```python
from build123d import *

# Parameters (mm, degrees)
SKETCH1_W                       = 344.6280001
SKETCH1_H                       = 182.714000078
BASE_FLANGE1_DEPTH              = 2.286
EDGE_FLANGE1_STRIP_W            = 13.9065
EDGE_FLANGE1_STRIP_H            = 2.286
EDGE_FLANGE1_STRIP_CUT_DEPTH    = 182.714000078
EDGE_FLANGE1_STRIP_2_W          = 13.9065
EDGE_FLANGE1_STRIP_2_H          = 2.286
EDGE_FLANGE1_STRIP_CUT_2_DEPTH  = 182.714000078
EDGE_FLANGE1_DEPTH              = 182.714000078
EDGE_FLANGE1_BEND_DEPTH         = 182.714000078
EDGE_FLANGE2_STRIP_W            = 13.9065
EDGE_FLANGE2_STRIP_H            = 2.286
EDGE_FLANGE2_STRIP_CUT_DEPTH    = 339.8655001
EDGE_FLANGE2_DEPTH              = 339.8655001
SKETCH17_W                      = 38.1
SKETCH17_H                      = 31.75
CUT_EXTRUDE1_DEPTH              = 200.412142834
FILLET1_R                       = 2.54
F_11_0_191_DIAMETER_HOLE1_D     = 4.8514
F_11_0_191_DIAMETER_HOLE1_DEPTH = 349.2000001
F_11_0_191_DIAMETER_HOLE1_TIP   = 1.457507604


# Sheet-metal steps are written as plain solids
with BuildPart() as part:
    # Sketch1 → Base-Flange1 (new body)
    with BuildSketch(Plane.XY):
        Rectangle(SKETCH1_W, SKETCH1_H)
    extrude(amount=-BASE_FLANGE1_DEPTH)

    # Edge-Flange1 strip (across the edge) → Edge-Flange1 strip cut (cut)
    with BuildSketch(Plane(origin=(172.31400005, -91.357000039, 0), x_dir=(-1, 0, 0), z_dir=(0, 1, 0))):
        with Locations((-4.572, -1.143)):
            Rectangle(EDGE_FLANGE1_STRIP_W, EDGE_FLANGE1_STRIP_H)
    extrude(amount=EDGE_FLANGE1_STRIP_CUT_DEPTH, mode=Mode.SUBTRACT)

    # Edge-Flange1 strip 2 (across the edge) → Edge-Flange1 strip cut 2 (cut)
    with BuildSketch(Plane(origin=(-172.31400005, 91.357000039, 0), x_dir=(1, 0, 0), z_dir=(0, -1, 0))):
        with Locations((-4.572, -1.143)):
            Rectangle(EDGE_FLANGE1_STRIP_2_W, EDGE_FLANGE1_STRIP_2_H)
    extrude(amount=EDGE_FLANGE1_STRIP_CUT_2_DEPTH, mode=Mode.SUBTRACT)

    # Edge-Flange1 section (across the edge) → Edge-Flange1 (add)
    with BuildSketch(Plane(origin=(172.31400005, -91.357000039, 0), x_dir=(-1, 0, 0), z_dir=(0, 1, 0))):
        with BuildLine():
            Line((-2.286, 2.38125), (-2.286, 20.32))
            Line((-2.286, 20.32), (0, 20.32))
            Line((0, 20.32), (0, 2.38125))
            ThreePointArc((0, 2.38125), (0.697451977, 0.697451977), (2.38125, 0))
            Line((2.38125, 0), (2.38125, -2.286))
            ThreePointArc((2.38125, -2.286), (-0.918994124, -0.918994124), (-2.286, 2.38125))
        make_face()
    extrude(amount=EDGE_FLANGE1_DEPTH)

    # Edge-Flange1 section 2 (across the edge) → Edge-Flange1 bend (add)
    with BuildSketch(Plane(origin=(-172.31400005, 91.357000039, 0), x_dir=(1, 0, 0), z_dir=(0, -1, 0))):
        with BuildLine():
            Line((-2.286, 2.38125), (-2.286, 20.32))
            Line((-2.286, 20.32), (0, 20.32))
            Line((0, 20.32), (0, 2.38125))
            ThreePointArc((0, 2.38125), (0.697451977, 0.697451977), (2.38125, 0))
            Line((2.38125, 0), (2.38125, -2.286))
            ThreePointArc((2.38125, -2.286), (-0.918994124, -0.918994124), (-2.286, 2.38125))
        make_face()
    extrude(amount=EDGE_FLANGE1_BEND_DEPTH)

    # Edge-Flange2 strip (across the edge) → Edge-Flange2 strip cut (cut)
    with BuildSketch(Plane(origin=(169.93275005, -91.357000039, -2.286), x_dir=(0, 1, 0), z_dir=(-1, 0, 0))):
        with Locations((-4.572, -1.143)):
            Rectangle(EDGE_FLANGE2_STRIP_W, EDGE_FLANGE2_STRIP_H)
    extrude(amount=EDGE_FLANGE2_STRIP_CUT_DEPTH, mode=Mode.SUBTRACT)

    # Edge-Flange2 section (across the edge) → Edge-Flange2 (add)
    with BuildSketch(Plane(origin=(169.93275005, -91.357000039, -2.286), x_dir=(0, 1, 0), z_dir=(-1, 0, 0))):
        with BuildLine():
            Line((-2.286, 2.38125), (-2.286, 19.05))
            Line((-2.286, 19.05), (0, 19.05))
            Line((0, 19.05), (0, 2.38125))
            ThreePointArc((0, 2.38125), (0.697451977, 0.697451977), (2.38125, 0))
            Line((2.38125, 0), (2.38125, -2.286))
            ThreePointArc((2.38125, -2.286), (-0.918994124, -0.918994124), (-2.286, 2.38125))
        make_face()
    extrude(amount=EDGE_FLANGE2_DEPTH)

    # Sketch17 → Cut-Extrude1 (cut, through all)
    with BuildSketch(Plane(origin=(0, 0, -2.286), x_dir=(-1, 0, 0), z_dir=(0, 0, -1))):
        with Locations((145.80275005, 75.482000039)):
            Rectangle(SKETCH17_W, SKETCH17_H)
    extrude(amount=-CUT_EXTRUDE1_DEPTH, mode=Mode.SUBTRACT)

    # Fillet1
    fillet1_edges = [part.edges().sort_by_distance(p)[0] for p in [
        (169.93275005, -92.500000039, -21.336),
        (-169.93275005, -92.500000039, -21.336),
        (-126.75275005, 91.357000039, -1.143),
        (-164.85275005, 91.357000039, -1.143),
        (-164.85275005, 59.607000039, -1.143),
        (-126.75275005, 59.607000039, -1.143),
        (173.45700005, -91.357000039, 20.32),
        (173.45700005, 91.357000039, 20.32),
        (-173.45700005, 91.357000039, 20.32),
        (-173.45700005, -91.357000039, 20.32),
    ]]
    fillet(fillet1_edges, radius=FILLET1_R)

    # #11 (0.191) Diameter Hole1
    with Locations(Plane.ZY.offset(174.60000005)):
        with Locations((10.080625, -73.742999961), (10.080625, 78.657000039), (10.080625, 53.257000039), (10.080625, 27.857000039), (10.080625, 2.457000039), (10.080625, -22.942999961), (10.080625, -48.342999961)):
            Hole(F_11_0_191_DIAMETER_HOLE1_D / 2, depth=F_11_0_191_DIAMETER_HOLE1_DEPTH)
            with Locations((0, 0, -(F_11_0_191_DIAMETER_HOLE1_DEPTH + F_11_0_191_DIAMETER_HOLE1_TIP / 2))):  # 118° drill point
                Cone(0, F_11_0_191_DIAMETER_HOLE1_D / 2, F_11_0_191_DIAMETER_HOLE1_TIP, mode=Mode.SUBTRACT)


solid = part.part
```
Can you work these out from the model? Positions are in its coordinate system, mm. A direction names the side the tool comes from. Round coordinates to 2 decimals unless told otherwise and drop trailing zeros. Loops run counter-clockwise (first coordinate to the right, second up) from the corner with the lowest first, then second, coordinate; pieces in that order, holes last. Notation, with made-up numbers: M -39,49 L 13,49 A34 cw 13,80 Z; hole C -29.75,85.5 d2. An arc over 180 degrees is marked long. Write item = value, one per line. Start each with the question number.
(1) Suppose I cut it at B-B on x = 34. Write out the boundary of the cut face in (y, z), plus the area to 3 significant figures.
(2) If we mould it in two halves opening along X, with no side actions, what happens to faces 4 (the face through (-172.314, 1, 13)), 5 (the face through (-174.6, 1, 13)), 6 (the face through (174.6, -1, 11))? For each: released by +X, released by -X, zero draft, split by the parting line, or undercut.
(3) I need wall thicknesses on line 1 along X through (y, z) = (71, 7.5); line 2 along Z through (x, y) = (-147, 5); line 3 along X through (y, z) = (-10, 0.5). Which ranges of each line are inside material? Lowest first, please.
(4) Suppose I cut it at C-C on y = -12. Write out the boundary of the cut face in (x, z), plus the area to 3 significant figures.
(5) I'm going to push flat-ended pins straight in: P1, Ø8, axis at y = -22.94, z = 10.08, coming from the -X side; P2, Ø0.5, axis at y = -90.5, z = -0.5, coming from the +X side; P3, Ø4, axis at x = 105, y = 10.5, coming from the +Z side; P4, Ø12, axis at x = -118.5, y = 32, coming from the -Z side. Where does each tip first touch, or does it pass through?
(6) Suppose I cut it at D-D on z = -15.5. Write out the boundary of the cut face in (x, y).
(7) Suppose I cut it at A-A on y = 69. Write out the boundary of the cut face in (x, z), plus the area to 3 significant figures.
(8) Which directions (+Z, -Z, +X, -X, +Y, -Y) give clear straight access to the entire face, cutting with the end or side of a thin tool? Please do faces 1 (the face through (172.314, -1, 11)), 2 (the face through (26, 91.357, -1)), 3 (the face through (2, -91.357, -13)).
Answer block:
q1.outline = M -93.64,-21.34 L -91.36,-21.34 L -91.36,-4.67 A2.38 cw -88.98,-2.29 L 91.36,-2.29 L 91.36,0 L -88.98,0 A4.67 ccw -93.64,-4.67 Z
q1.area = 463 mm²
q2.face_4 = undercut
q2.face_5 = released by -X
q2.face_6 = released by +X
q3.line_1 = -174.6 to -172.31, 172.31 to 174.6
q3.line_2 = -2.29 to 0
q3.line_3 = -174.2 to -171.39, 171.39 to 174.2
q4.outline = M -174.6,2.38 A4.67 ccw -169.93,-2.29 L 169.93,-2.29 A4.67 ccw 174.6,2.38 L 174.6,20.32 L 172.31,20.32 L 172.31,2.38 A2.38 cw 169.93,0 L -169.93,0 A2.38 cw -172.31,2.38 L -172.31,20.32 L -174.6,20.32 Z
q4.area = 884 mm²
q5.P1 = -174.6
q5.P2 = 173.79
q5.P3 = 0
q5.P4 = -2.29
q6.outline = M -169.93,-93.64 L 169.93,-93.64 L 169.93,-91.36 L -169.93,-91.36 Z
q7.outline = M -174.6,2.38 A4.67 ccw -169.93,-2.29 L -164.85,-2.29 L -164.85,0 L -169.93,0 A2.38 cw -172.31,2.38 L -172.31,20.32 L -174.6,20.32 Z; M -126.75,-2.29 L 169.93,-2.29 A4.67 ccw 174.6,2.38 L 174.6,20.32 L 172.31,20.32 L 172.31,2.38 A2.38 cw 169.93,0 L -126.75,0 Z
q7.area = 797 mm²
q8.face_1 = +Z, +Y, -Y
q8.face_2 = +Z, -Z, +X, -X, +Y
q8.face_3 = -Z, +X, -X, +Y
